For this review, take the finished solid that the model builds, in its own axes (mm). A direction names the side the tool comes from. Round coordinates to 2 decimals unless told otherwise and drop trailing zeros. Write each loop counter-clockwise with the first axis right and the second up, starting at its lowest first coordinate (ties: lowest second). Pieces come first, ordered by that corner, then holes. Notation, with made-up numbers: (64.5, 41.25) -> (90.5, 41.25) arc R11 cw to (90.5, 51.25) -> close; hole circle Ø2 at (-4.75, 75.5). An arc over 180 degrees is marked (long way). Write each question's results on one line, items separated by ' | '. Start each with the question number.
Item 1: Add section B-B (y = -16). State the section outline as (x, z) points, plus the area to 3 significant figures.
Item 2: To check wall thickness, follow line 1 along X through (y, z) = (16, 6.25); line 2 along X through (y, z) = (24, 4); line 3 along Z through (x, y) = (-10.5, 12.5). State the ranges of each line that lie inside material, in increasing order.
Item 3: Tool access review of faces 1 (the flat face through (-5.68, 21.9, 3.41)), 2 (the cylindrical face through (-0.195, 22.513, 3.944)), 3 (the cylindrical face through (7.675, -14.536, 1.548)): name each direction out of +Z, -Z, +X, -X, +Y, -Y from which nothing blocks a thin tool from reaching the whole face with its end or side.
Item 4: Add section C-C (y = 16). State the section outline as (x, z) points, plus the area to 3 significant figures.
Item 5: Add section D-D (x = -8). State the section outline as (y, z) points, plus the area to 3 significant figures.
Item 6: Add section A-A (x = 0). State the section outline as (y, z) points.
Item 7: Clearance check with flat-ended pins moving along their axes: pin 1 (1.8 mm diameter, centred on x = 8, y = 16, fed in from +Z); pin 2 (2.5 mm diameter, centred on x = 8, y = -16, fed in from +Z); pin 3 (1.8 mm diameter, centred on x = 0, y = 24, fed in from -Z); pin 4 (1.5 mm diameter, centred on x = 0, y = -13, fed in from +Z). State where each tip first meets the part, or that it passes through.
Item 8: The part is to be moulded in two halves that separate along X. For faces 4 (the flat face through (-0.224, -0.045, 5.635)), 5 (the cylindrical face through (7.088, 10.657, 4.518)), 6 (the flat face through (-16, 8, 4)), say which applies: +X half, -X half, draft (parallel to the pull), parting line (faces both ways), or undercut.
from build123d import *

# Parameters (mm, degrees)
F0_W     = 32
F0_H     = 64
F1_ANGLE = 10
F2_R     = 1.5
F3_DEPTH = 6
F4_R     = 1.5
F5_DEPTH = 8


with BuildPart() as f1:
    # F0 (on Top) → F1 (revolve)
    with BuildSketch(Plane.XY):
        Rectangle(F0_W, F0_H)
    revolve(axis=Axis((0, -32, 0), (1, 0, 0)), revolution_arc=F1_ANGLE)

    # F2 (on face) → F3 (cut)
    with BuildSketch(Plane(origin=(0, -0.9649180674, 5.4723222932), x_dir=(1, 0, 0), z_dir=(0, -0.1736481777, 0.984807753))):
        with Locations((-5.6568542495, 22.1430061531)):
            Circle(F2_R)
        with Locations((5.6568542495, 22.1430061531)):
            Circle(F2_R)
        with Locations((5.6568542495, 10.8292976541)):
            Circle(F2_R)
        with Locations((-5.6568542495, 10.8292976541)):
            Circle(F2_R)
    extrude(amount=-F3_DEPTH, mode=Mode.SUBTRACT)

    # F4 (on face) → F5 (cut)
    with BuildSketch(Plane(origin=(0, 0, 0), x_dir=(1, 0, 0), z_dir=(0, 0, -1))):
        with Locations((0, -8)):
            Circle(F4_R)
        with Locations((8, -16)):
            Circle(F4_R)
        with Locations((0, -24)):
            Circle(F4_R)
        with Locations((-8, -16)):
            Circle(F4_R)
        with Locations((-8, 16)):
            Circle(F4_R)
        with Locations((8, 16)):
            Circle(F4_R)
    extrude(amount=-F5_DEPTH, mode=Mode.SUBTRACT)


solid = f1.part
Responses:
1) outline: (-16, 0) -> (-9.5, 0) -> (-9.5, 2.82) -> (-16, 2.82) -> close; (-6.5, 0) -> (6.5, 0) -> (6.5, 2.82) -> (-6.5, 2.82) -> close; (9.5, 0) -> (16, 0) -> (16, 2.82) -> (9.5, 2.82) -> close | area: 73.4 mm^2
2) line 1: x = -16 to -9.5, -6.5 to 6.5, 9.5 to 16 | line 2: x = -16 to -1.5, 1.5 to 16 | line 3: z = 0 to 7.85
3) face 1: none | face 2: -Z | face 3: +Z, -Z
4) outline: (-16, 0) -> (-9.5, 0) -> (-9.5, 8) -> (-6.5, 8) -> (-6.5, 0) -> (6.5, 0) -> (6.5, 8) -> (9.5, 8) -> (9.5, 0) -> (16, 0) -> (16, 8.46) -> (-16, 8.46) -> close | area: 223 mm^2
5) outline: (-32, 0) -> (-17.5, 0) -> (-17.5, 2.56) -> close; (-14.5, 0) -> (14.5, 0) -> (14.5, 8) -> (17.5, 8) -> (17.5, 0) -> (32, 0) arc R64 ccw to (31.03, 11.11) -> (-14.5, 3.09) -> close | area: 325 mm^2
6) outline: (-32, 0) -> (6.5, 0) -> (6.5, 6.79) -> close; (9.5, 0) -> (22.5, 0) -> (22.5, 8) -> (25.5, 8) -> (25.5, 0) -> (32, 0) arc R64 ccw to (31.03, 11.11) -> (9.5, 7.32) -> close
7) pin 1: stops at z = 8.62 | pin 2: passes through | pin 3: stops at z = 8 | pin 4: stops at z = 3.48
8) face 4: draft | face 5: undercut | face 6: -X half
